from build123d import *

# Parameters (mm, degrees)
SKETCH_3_R           = 9.5
CUT_EXTRUDE_1_DEPTH  = 321.526909947
SKETCH_4_R           = 9.5
CUT_EXTRUDE_2_DEPTH  = 321.526909947
SKETCH_5_R           = 9.5
CUT_EXTRUDE_3_DEPTH  = 321.526909947
SKETCH_6_R           = 9.5
CUT_EXTRUDE_4_DEPTH  = 321.526909947
SKETCH_7_R           = 9.5
CUT_EXTRUDE_5_DEPTH  = 321.526909947
SKETCH_8_R           = 9.5
CUT_EXTRUDE_6_DEPTH  = 321.526909947
SKETCH_9_R           = 9.5
CUT_EXTRUDE_7_DEPTH  = 321.526909947
SKETCH_10_R          = 9.5
CUT_EXTRUDE_8_DEPTH  = 321.526909947
SKETCH_11_R          = 9.5
CUT_EXTRUDE_9_DEPTH  = 321.526909947
SKETCH_12_R          = 9.5
CUT_EXTRUDE_10_DEPTH = 321.526909947
SKETCH_13_R          = 9.5
CUT_EXTRUDE_11_DEPTH = 321.526909947
SKETCH_14_R          = 9.5
CUT_EXTRUDE_12_DEPTH = 321.526909947


with BuildPart() as part:
    # Эскиз1 → Повернуть1 (revolve)
    with BuildSketch(Plane.XY, mode=Mode.PRIVATE) as revolve_1_sk:
        Polygon((0, 0), (265, 0), (265, 127.5), (239, 127.5), (239, 100), (239, 95), (220, 95), (220, 94), (200, 94), (144, 65.5), (70, 65.5), (25, 41), (1.5, 41), (3, 45), (0, 45), align=None)
    revolve(revolve_1_sk.sketch.rotate(Axis((0, 0, 0), (1, 0, 0)), 90), axis=Axis((0, 0, 0), (1, 0, 0)))

    # Эскиз2 → Вырез-Повернуть1 (revolve, cut)
    with BuildSketch(Plane.XY, mode=Mode.PRIVATE) as cut_revolve_1_sk:
        with BuildLine():
            Line((0, 0), (257, 0))
            Line((257, 0), (257, 34))
            Line((257, 34), (239, 34))
            Line((239, 34), (226, 47))
            Line((226, 47), (203.5, 47))
            Line((203.5, 47), (203.5, 55))
            Line((203.5, 55), (147.669872, 55))
            ThreePointArc((147.669872, 55), (146.273624348, 54.108499061), (146.669872, 52.5))
            Line((146.669872, 52.5), (143.5, 52.5))
            ThreePointArc((143.5, 52.5), (142.75, 52.602347572), (142, 52.5))
            Line((142, 52.5), (90, 52.5))
            ThreePointArc((90, 52.5), (79.13262933, 46.740617582), (70, 38.502577))
            Line((70, 38.502577), (42, 31))
            Line((42, 31), (0, 31))
            Line((0, 31), (0, 0))
        make_face()
    revolve(cut_revolve_1_sk.sketch.rotate(Axis((0, 0, 0), (1, 0, 0)), 90), axis=Axis((0, 0, 0), (1, 0, 0)), mode=Mode.SUBTRACT)

    # Эскиз3 → Вырез-Вытянуть1 (cut, through all)
    with BuildSketch(Plane(origin=(0, 0, 0), x_dir=(0, 0, -1), z_dir=(1, 0, 0))):
        with Locations((0, 113)):
            Circle(SKETCH_3_R)
    extrude(amount=CUT_EXTRUDE_1_DEPTH, mode=Mode.SUBTRACT)

    # Эскиз4 → Вырез-Вытянуть2 (cut, through all)
    with BuildSketch(Plane(origin=(0, 0, 0), x_dir=(0, 0, -1), z_dir=(1, 0, 0))):
        with Locations((-56.5, 97.860870628)):
            Circle(SKETCH_4_R)
    extrude(amount=CUT_EXTRUDE_2_DEPTH, mode=Mode.SUBTRACT)

    # Эскиз5 → Вырез-Вытянуть3 (cut, through all)
    with BuildSketch(Plane(origin=(0, 0, 0), x_dir=(0, 0, -1), z_dir=(1, 0, 0))):
        with Locations((-97.860870628, 56.5)):
            Circle(SKETCH_5_R)
    extrude(amount=CUT_EXTRUDE_3_DEPTH, mode=Mode.SUBTRACT)

    # Эскиз6 → Вырез-Вытянуть4 (cut, through all)
    with BuildSketch(Plane(origin=(0, 0, 0), x_dir=(0, 0, -1), z_dir=(1, 0, 0))):
        with Locations((-113, 0)):
            Circle(SKETCH_6_R)
    extrude(amount=CUT_EXTRUDE_4_DEPTH, mode=Mode.SUBTRACT)

    # Эскиз7 → Вырез-Вытянуть5 (cut, through all)
    with BuildSketch(Plane(origin=(0, 0, 0), x_dir=(0, 0, -1), z_dir=(1, 0, 0))):
        with Locations((-97.860870628, -56.5)):
            Circle(SKETCH_7_R)
    extrude(amount=CUT_EXTRUDE_5_DEPTH, mode=Mode.SUBTRACT)

    # Эскиз8 → Вырез-Вытянуть6 (cut, through all)
    with BuildSketch(Plane(origin=(0, 0, 0), x_dir=(0, 0, -1), z_dir=(1, 0, 0))):
        with Locations((-56.5, -97.860870628)):
            Circle(SKETCH_8_R)
    extrude(amount=CUT_EXTRUDE_6_DEPTH, mode=Mode.SUBTRACT)

    # Эскиз9 → Вырез-Вытянуть7 (cut, through all)
    with BuildSketch(Plane(origin=(0, 0, 0), x_dir=(0, 0, -1), z_dir=(1, 0, 0))):
        with Locations((0, -113)):
            Circle(SKETCH_9_R)
    extrude(amount=CUT_EXTRUDE_7_DEPTH, mode=Mode.SUBTRACT)

    # Эскиз10 → Вырез-Вытянуть8 (cut, through all)
    with BuildSketch(Plane(origin=(0, 0, 0), x_dir=(0, 0, -1), z_dir=(1, 0, 0))):
        with Locations((56.5, -97.860870628)):
            Circle(SKETCH_10_R)
    extrude(amount=CUT_EXTRUDE_8_DEPTH, mode=Mode.SUBTRACT)

    # Эскиз11 → Вырез-Вытянуть9 (cut, through all)
    with BuildSketch(Plane(origin=(0, 0, 0), x_dir=(0, 0, -1), z_dir=(1, 0, 0))):
        with Locations((97.860870628, -56.5)):
            Circle(SKETCH_11_R)
    extrude(amount=CUT_EXTRUDE_9_DEPTH, mode=Mode.SUBTRACT)

    # Эскиз12 → Вырез-Вытянуть10 (cut, through all)
    with BuildSketch(Plane(origin=(0, 0, 0), x_dir=(0, 0, -1), z_dir=(1, 0, 0))):
        with Locations((113, 0)):
            Circle(SKETCH_12_R)
    extrude(amount=CUT_EXTRUDE_10_DEPTH, mode=Mode.SUBTRACT)

    # Эскиз13 → Вырез-Вытянуть11 (cut, through all)
    with BuildSketch(Plane(origin=(0, 0, 0), x_dir=(0, 0, -1), z_dir=(1, 0, 0))):
        with Locations((97.860870628, 56.5)):
            Circle(SKETCH_13_R)
    extrude(amount=CUT_EXTRUDE_11_DEPTH, mode=Mode.SUBTRACT)

    # Эскиз14 → Вырез-Вытянуть12 (cut, through all)
    with BuildSketch(Plane(origin=(0, 0, 0), x_dir=(0, 0, -1), z_dir=(1, 0, 0))):
        with Locations((56.5, 97.860870628)):
            Circle(SKETCH_14_R)
    extrude(amount=CUT_EXTRUDE_12_DEPTH, mode=Mode.SUBTRACT)


solid = part.part
Here's how the part is built. I have some questions about the finished solid (model axes, mm). A direction names the side the tool comes from. Round coordinates to 2 decimals unless told otherwise and drop trailing zeros. Loops run counter-clockwise (first coordinate to the right, second up) from the corner with the lowest first, then second, coordinate; pieces in that order, holes last.
1. If we section it at D-D on z = 0: Count the separate pieces of the cut face and the enclosed holes in it, plus the area to 3 significant figures.
Answer list:
separate pieces: 3
enclosed holes: 0
area: 15,500 mm2
2. If we section it at C-C on x = 213: Write out the boundary of the cut face in (y, z), plus the area to 3 significant figures.
Answer list:
outline: circle Ø188 at (0, 0); hole circle Ø94 at (0, 0)
area: 20,800 mm2
3. We'd pull the mould along Z, two halves only. Please class faces 4 (the face through (0, -10.6, 29.4)), 5 (the face through (251.818, -95.007, 47.439)), 6 (the face through (27.185, 41.186, -9.146)): +Z half, -Z half, draft (parallel to the pull), parting line (faces both ways), or undercut.
Answer list:
face 4: draft
face 5: undercut
face 6: parting line
4. If we section it at A-A on y = -113: Write out the boundary of the cut face in (x, z).
Answer list:
outline: (239, -59.05) - (265, -59.05) - (265, -9.5) - (239, -9.5) - close; (239, 9.5) - (265, 9.5) - (265, 59.05) - (239, 59.05) - close
5. For P1, Ø10, axis at x = 40.5, z = 11.5, coming from the -Y side; P2, Ø10, axis at x = 36, y = -19.5, coming from the +Z side; P3, Ø4, axis at x = 58, z = 10, coming from the -Y side, each with a flat end and sliding along its axis, tell me the tip position at first contact or that it passes through.
Answer list:
P1: stops at y = -51.07
P2: stops at z = 46.33
P3: stops at y = -59.26
6. Which directions (+Z, -Z, +X, -X, +Y, -Y) give clear straight access to the entire face, cutting with the end or side of a thin tool? Please do faces 1 (the face through (1.479, 39.923, 20.765)), 2 (the face through (251.818, 100.714, -65.561)), 3 (the face through (203.5, -25, -40)).
Answer list:
face 1: -X
face 2: +X, -X
face 3: none
7. If I drill on line 1 along Y through (x, z) = (256, 0); line 2 along X through (y, z) = (39, -117); line 3 along Y through (x, z) = (186, 38.5), over which ranges is the centre line in solid material (lowest first)?
Answer list:
line 1: y = -127.5 to -122.5, -103.5 to -34, 34 to 103.5, 122.5 to 127.5
line 2: x = 239 to 265
line 3: y = -77.88 to -39.28, 39.28 to 77.88
